Geometry: final body of the model. Coordinates: model frame, mm. Face numbers are marked on the shaded views. A direction names the side the tool comes from. Round coordinates to 2 decimals unless told otherwise and drop trailing zeros. Order: outer loops, then holes, each group sorted by start corner. A loop starts at its lowest first (then second) coordinate and runs counter-clockwise, first axis right, second up. Notation, with made-up numbers: (-14.75, 84) - (-8.75, 84) arc R14 ccw to (-8.75, 105) - close; hole circle Ø2 at (1, 77.5). An arc over 180 degrees is marked (long way). Put each result on its own line as item: value. Start each with the question number.
(1) Pin query (flat end, axial travel): P1, Ø1, axis at y = 12, z = -12.5, coming from the +X side; P2, Ø1.5, axis at x = -0.5, z = 6, coming from the +Y side; P3, Ø1.6, axis at x = 17.5, y = 12, coming from the -Z side. Return the tip coordinate at first contact, or that it passes through.
(2) Access query for the marked faces 4, 5, 6 and 7. Directions: +Z, -Z, +X, -X, +Y, -Y. A direction counts if a zero-diameter tool reaches every point of the face in a straight line with its end or side. Return the directions, or none.
(3) Section B-B (x = -2). Output: boundary loops of the cut face in (y, z).
(4) Section D-D (z = 5.25). Count the separate pieces of the cut face and the enclosed holes in it, and give its area (3 significant figures).
(5) Section A-A (y = 5). Output: boundary loops of the cut face in (x, z).
(6) Material intervals for L1, parallel to Z at x = 8.5, y = 1.75; L2, parallel to X at y = -3, z = 2; L3, parallel to X at y = 2, z = -5.5, sorted ascending. Write a range as [from, to].
(7) Pull-direction query (Z, two-part tool) for the marked faces 1, 2 and 3; classes: released by +Z, released by -Z, zero draft, split by the parting line, or undercut.
(8) Section C-C (y = 10.75). Output: boundary loops of the cut face in (x, z), and give its area (3 significant figures).
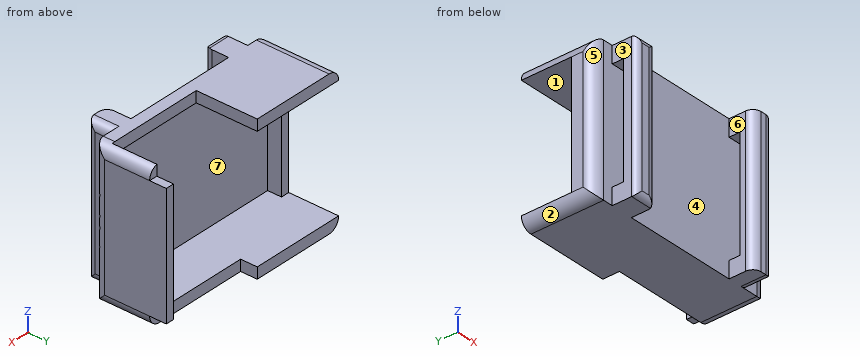
from build123d import *

# Parameters (mm, degrees)
SKETCH_1_W          = 36
SKETCH_1_H          = 26
EXTRUDE_1_DEPTH     = 14.6
SKETCH_2_W          = 33
SKETCH_2_H          = 22
CUT_EXTRUDE_1_DEPTH = 13
SKETCH_3_W          = 36
SKETCH_3_H          = 26
CUT_EXTRUDE_2_DEPTH = 4.5
SKETCH_4_W          = 1.5
SKETCH_4_H          = 22
CUT_EXTRUDE_3_DEPTH = 6
SKETCH_7_W          = 17
SKETCH_7_H          = 2
SKETCH_7_W_2        = 1.5
SKETCH_7_H_2        = 22
EXTRUDE_4_DEPTH     = 3
SKETCH_5_W          = 4
SKETCH_5_H          = 3
EXTRUDE_5_DEPTH     = 2
SKETCH_8_W          = 4
SKETCH_8_H          = 26
EXTRUDE_6_DEPTH     = 2.5
SKETCH_10_W         = 17.5
SKETCH_10_H         = 2
CUT_EXTRUDE_4_DEPTH = 8
FILLET_2_R          = 1
FILLET_3_R          = 1.5
FILLET_4_R          = 1.5
FILLET_5_R          = 1.5
FILLET_6_R          = 2
FILLET_7_R          = 2
FILLET_8_R          = 2
FILLET_START        = -14
FILLET_9_DEPTH      = 28


with BuildPart() as part:
    # 草图1 → 凸台-拉伸1 (new body)
    with BuildSketch(Plane(origin=(0, 0, 0), x_dir=(1, 0, 0), z_dir=(0, 1, 0))):
        Rectangle(SKETCH_1_W, SKETCH_1_H)
    extrude(amount=EXTRUDE_1_DEPTH)

    # 草图2 → 切除-拉伸1 (cut)
    with BuildSketch(Plane(origin=(0, 14.6, 0), x_dir=(1, 0, 0), z_dir=(0, 1, 0))):
        Rectangle(SKETCH_2_W, SKETCH_2_H)
    extrude(amount=-CUT_EXTRUDE_1_DEPTH, mode=Mode.SUBTRACT)

    # 草图3 → 切除-拉伸2 (cut)
    with BuildSketch(Plane(origin=(0, 14.6, 0), x_dir=(1, 0, 0), z_dir=(0, 1, 0))):
        Rectangle(SKETCH_3_W, SKETCH_3_H)
    extrude(amount=-CUT_EXTRUDE_2_DEPTH, mode=Mode.SUBTRACT)

    # 草图4 → 切除-拉伸3 (cut)
    with BuildSketch(Plane(origin=(0, 10.1, 0), x_dir=(1, 0, 0), z_dir=(0, 1, 0))):
        with Locations((-17.25, 0)):
            Rectangle(SKETCH_4_W, SKETCH_4_H)
    extrude(amount=-CUT_EXTRUDE_3_DEPTH, mode=Mode.SUBTRACT)

    # 草图7 → 凸台-拉伸4 (add)
    with BuildSketch(Plane(origin=(0, 10.1, 0), x_dir=(1, 0, 0), z_dir=(0, 1, 0))):
        with Locations((-9.5, 12)):
            Rectangle(SKETCH_7_W, SKETCH_7_H)
        with Locations((-9.5, -12)):
            Rectangle(SKETCH_7_W, SKETCH_7_H)
        with Locations((17.25, 0)):
            Rectangle(SKETCH_7_W_2, SKETCH_7_H_2)
    extrude(amount=EXTRUDE_4_DEPTH)

    # 草图5 → 凸台-拉伸5 (add)
    with BuildSketch(Plane(origin=(0, 0, 0), x_dir=(-1, 0, 0), z_dir=(0, -1, 0))):
        with Locations((-12.2, -11.5)):
            Rectangle(SKETCH_5_W, SKETCH_5_H)
        with Locations((12.2, -11.5)):
            Rectangle(SKETCH_5_W, SKETCH_5_H)
        with Locations((-12.2, 11.5)):
            Rectangle(SKETCH_5_W, SKETCH_5_H)
        with Locations((12.2, 11.5)):
            Rectangle(SKETCH_5_W, SKETCH_5_H)
    extrude(amount=EXTRUDE_5_DEPTH)

    # 草图8 → 凸台-拉伸6 (add)
    with BuildSketch(Plane(origin=(0, -2, 0), x_dir=(-1, 0, 0), z_dir=(0, -1, 0))):
        with Locations((-12.2, 0)):
            Rectangle(SKETCH_8_W, SKETCH_8_H)
        with Locations((12.2, 0)):
            Rectangle(SKETCH_8_W, SKETCH_8_H)
    extrude(amount=EXTRUDE_6_DEPTH)

    # 草图10 → 切除-拉伸4 (cut)
    with BuildSketch(Plane(origin=(0, 10.1, 0), x_dir=(1, 0, 0), z_dir=(0, 1, 0))):
        with Locations((7.75, -12)):
            Rectangle(SKETCH_10_W, SKETCH_10_H)
    extrude(amount=-CUT_EXTRUDE_4_DEPTH, mode=Mode.SUBTRACT)

    # 圆角2
    fillet_2_edges = [part.edges().sort_by_distance(p)[0] for p in [
        (-14.2, -4.5, 0),
        (-12.2, -4.5, -13),
        (-12.2, -4.5, 13),
    ]]
    fillet(fillet_2_edges, radius=FILLET_2_R)

    # 圆角3
    fillet_3_edges = [part.edges().sort_by_distance(p)[0] for p in [
        (14.2, -2.25, 13),
        (14.2, -2.25, -13),
        (14.2, -4.5, 0),
    ]]
    fillet(fillet_3_edges, radius=FILLET_3_R)

    # 圆角4
    fillet_4_edges = [part.edges().sort_by_distance(p)[0] for p in [
        (10.2, -4.5, 0),
    ]]
    fillet(fillet_4_edges, radius=FILLET_4_R)

    # 圆角5
    # the kernel refuses this fillet: 1.5 mm, written as the material it takes off along each edge
    with BuildSketch(Plane(origin=(-10.2, -4.5, 15.75), x_dir=(0, 1, 0), z_dir=(0, 0, -1))) as fillet_5_piece_1:
        with BuildLine():
            CenterArc((FILLET_5_R, -FILLET_5_R), FILLET_5_R, 90, 90)
            Line((0, -FILLET_5_R), (0, 0))
            Line((0, 0), (FILLET_5_R, 0))
        make_face()
    extrude(amount=31.5, mode=Mode.SUBTRACT)

    # 圆角6
    fillet_6_edges = [part.edges().sort_by_distance(p)[0] for p in [
        (-18, 6.55, 13),
        (-18, 6.55, -13),
        (-18, 0, 0),
    ]]
    fillet(fillet_6_edges, radius=FILLET_6_R)

    # 圆角7
    fillet_7_edges = [part.edges().sort_by_distance(p)[0] for p in [
        (18, 5.05, -13),
    ]]
    fillet(fillet_7_edges, radius=FILLET_7_R)

    # 圆角8
    fillet_8_edges = [part.edges().sort_by_distance(p)[0] for p in [
        (18, 5.05, 13),
    ]]
    fillet(fillet_8_edges, radius=FILLET_8_R)

    # 圆角9: read off the stored shape, not the designer's step
    # 圆角9 outline → 圆角9 (cut)
    with BuildSketch(Plane.XY.offset(FILLET_START)):
        with BuildLine():
            Line((18, 0), (18, 2))
            add(Edge.make_bspline(
                [(18, 2), (18, 0), (16, 0)],
                knots=[0, 0, 0, 1, 1, 1], degree=2, weights=[1, 0.707106781, 1]))
            Line((16, 0), (18, 0))
        make_face()
    extrude(amount=FILLET_9_DEPTH, mode=Mode.SUBTRACT)


solid = part.part
Checks:
1. P1: stops at x = -1
1. P2: stops at y = 1.6
1. P3: stops at z = -11
2. face 4: none
2. face 5: +Z, -Z, -X, -Y
2. face 6: +Z, -Z, -Y
2. face 7: +Y
3. outline: (0, -13) - (13.1, -13) - (13.1, -11) - (1.6, -11) - (1.6, 11) - (13.1, 11) - (13.1, 13) - (0, 13) - close
4. separate pieces: 3
4. enclosed holes: 0
4. area: 95.2 mm²
5. outline: (-18, -11) arc R2 ccw to (-16, -13) - (16, -13) arc R2 ccw to (18, -11) - (18, 11) arc R2 ccw to (16.5, 12.94) - (16.5, -11) - close; (-18, 11) - (-1, 11) - (-1, 13) - (-16, 13) arc R2 ccw to start
6. L1: z = [-13, -11], [11, 13]
6. L2: x = [-14.2, -10.2], [10.2, 14.2]
6. L3: x = [-18, -16.5], [16.5, 18]
7. face 1: undercut
7. face 2: released by -Z
7. face 3: zero draft
8. outline: (-18, -11) arc R2 ccw to (-16, -13) - (-1, -13) - (-1, -11) - close; (-18, 11) - (-1, 11) - (-1, 13) - (-16, 13) arc R2 ccw to start; (16.5, -11) - (18, -11) - (18, 11) - (16.5, 11) - close
8. area: 99.3 mm²
